Check sheet for the drawn part. Datum: minimum x, y, z corner. Units: mm. Coordinates: 2 decimals unless noted, no trailing zeros. Write each loop counter-clockwise with the first axis right and the second up, starting at its lowest first coordinate (ties: lowest second). Pieces come first, ordered by that corner, then holes. Notation, with made-up numbers: (-28, -37) -> (-24, -37) arc R33 ccw to (-24, -3) -> close; hole circle Ø4 at (-17.5, 7.25). An arc over 180 degrees is marked (long way). Answer in a Markdown table with one row per item. Add a question column.
Q1. Gauge pin test, flat ends, axial feed: P1, Ø10, axis at y = 18.5, z = 23, coming from the -X side; P2, Ø12, axis at y = 14.5, z = 29, coming from the +X side; P3, Ø2, axis at x = 36.5, y = 16.5, coming from the +Z side; P4, Ø5, axis at x = 16, z = 5.5, coming from the -Y side. Record the tip position at first contact, or that the pin passes through.
Q2. Section check D-D, the plane z = 5. Record the boundary of the cut face in (x, y), and give its area (3 significant figures).
Q3. Thickness scan on line 1 (Z direction, x = 28, y = 19); line 2 (Z direction, x = 5, y = 26.2); line 3 (Y direction, x = 11, z = 32.5). Record the ranges inside material, lowest first.
Q4. Section check B-B, the plane z = 25. Record the boundary of the cut face in (x, y).
Q5. Release check for a two-part mould opening along X. For the marked faces 1, 2 and 3 record: pulls with the +X half, pulls with the -X half, needs draft (parallel to the pull), parting line crosses it, or undercut.
Q6. Section check A-A, the plane x = 28. Record the boundary of the cut face in (y, z).
Q7. Section check C-C, the plane y = 18. Record the boundary of the cut face in (x, z).
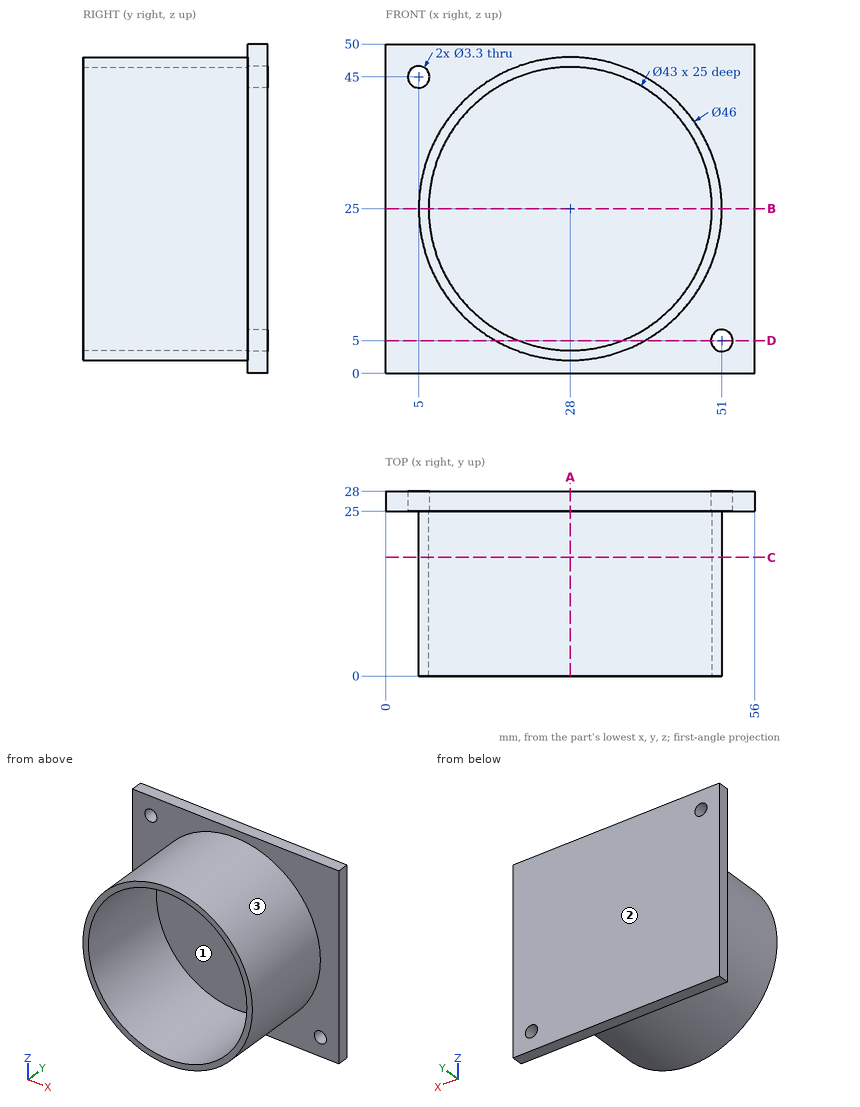
Calculated:
| question | item | result |
|---|---|---|
| 1 | P1 | stops at x = 5 |
| 1 | P2 | stops at x = 51 |
| 1 | P3 | stops at z = 46.74 |
| 1 | P4 | stops at y = 0 |
| 2 | outline | (0, 25) -> (16.64, 25) -> (16.64, 0) -> (20.11, 0) -> (20.11, 25) -> (35.89, 25) -> (35.89, 0) -> (39.36, 0) -> (39.36, 25) -> (49.35, 25) -> (49.35, 28) -> (0, 28) -> close; (52.65, 25) -> (56, 25) -> (56, 28) -> (52.65, 28) -> close |
| 2 | area | 331 mm² |
| 3 | line 1 | z = 2 to 3.5, 46.5 to 48 |
| 3 | line 2 | z = 0 to 43.35, 46.65 to 50 |
| 3 | line 3 | y = 25 to 28 |
| 4 | outline | (0, 25) -> (5, 25) -> (5, 0) -> (6.5, 0) -> (6.5, 25) -> (49.5, 25) -> (49.5, 0) -> (51, 0) -> (51, 25) -> (56, 25) -> (56, 28) -> (0, 28) -> close |
| 5 | face 1 | undercut |
| 5 | face 2 | needs draft |
| 5 | face 3 | parting line crosses it |
| 6 | outline | (0, 2) -> (25, 2) -> (25, 0) -> (28, 0) -> (28, 50) -> (25, 50) -> (25, 48) -> (0, 48) -> (0, 46.5) -> (25, 46.5) -> (25, 3.5) -> (0, 3.5) -> close |
| 7 | outline | circle Ø46 at (28, 25); hole circle Ø43 at (28, 25) |
